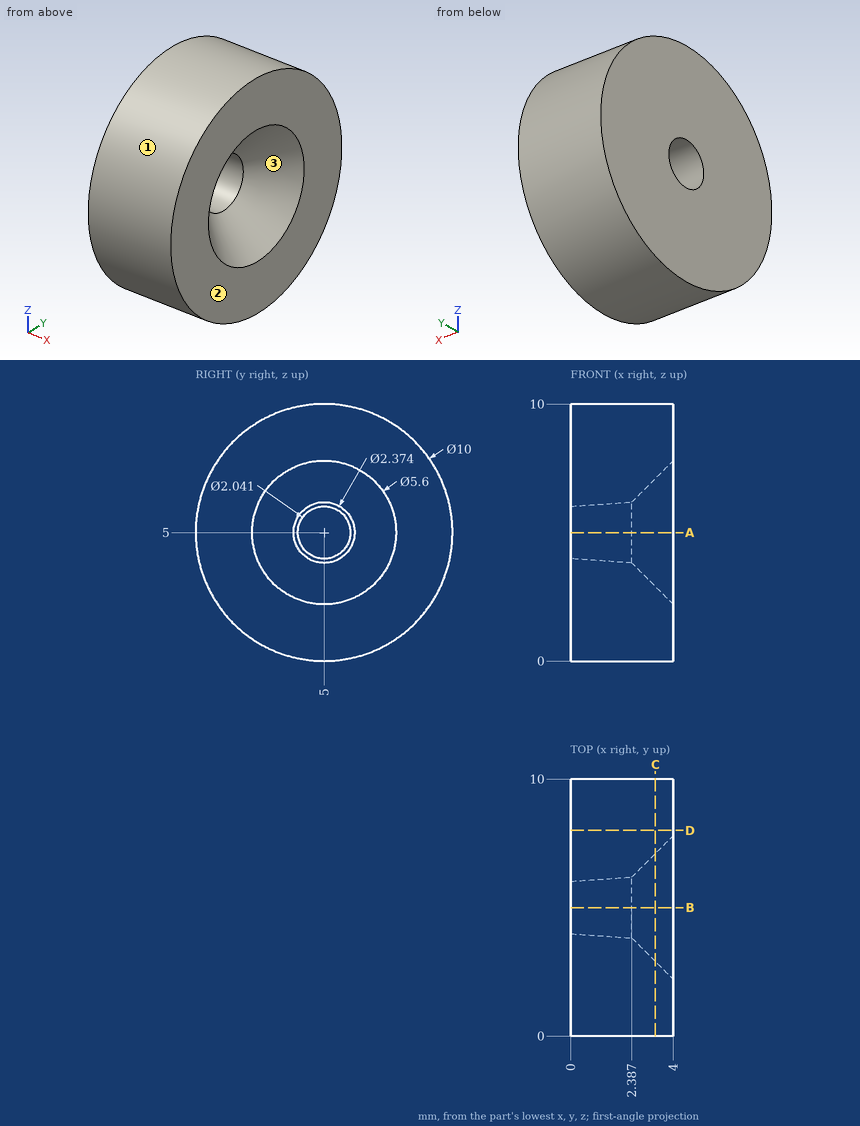
The drawing under review shows one solid part. Ordinate dimensions are in mm from its lowest x, y, z. Give positions to 0.01 mm unless a question says otherwise; leave off trailing zeros. Order: outer loops, then holes, each group sorted by start corner. A loop starts at its lowest first (then second) coordinate and runs counter-clockwise, first axis right, second up. Notation, with made-up numbers: (-23, 76) -> (1, 76) arc R35 ccw to (1, 111) -> close; hole circle Ø9 at (34, 5.5). An arc over 180 degrees is marked (long way). Write item = value, one per line. Start each with the question number.
(1) Mouldability with a two-part tool opening along Z and no side actions: class the marked faces 1, 2 and 3 as +Z half, -Z half, draft (parallel to the pull), parting line (faces both ways), or undercut.
(2) For pin 1 (1.5 mm diameter, centred on x = 1.5, y = 6.5, fed in from +Z), flat-tipped, find the tip position at first contact; note if it passes through.
(3) We need section D-D on y = 8. Write out the cut boundary in (x, z), plus the area to 3 significant figures.
(4) We need section C-C on x = 3.3. Write out the cut boundary in (y, z).
(5) To check wall thickness, follow line 1 along Z through (x, y) = (0.5, 5.5) (1 decimal); line 2 along Z through (x, y) = (3.7, 6.25) (1 decimal); line 3 along Y through (x, z) = (3.8, 3) (1 decimal). State the ranges of each line that lie inside material, in increasing order.
(6) We need section A-A on z = 5. Write out the cut boundary in (x, y), plus the area to 3 significant figures.
Numbers:
q1.face_1 = parting line
q1.face_2 = draft
q1.face_3 = undercut
q2.pin_1 = 9.94
q3.outline = (0, 1) -> (4, 1) -> (4, 9) -> (0, 9) -> close
q3.area = 32.0 mm^2
q4.outline = circle Ø10 at (5, 5); hole circle Ø4.2 at (5, 5)
q5.line_1 = 0 to 4.1, 5.9 to 10
q5.line_2 = 0.2 to 2.8, 7.2 to 9.8
q5.line_3 = 0.4 to 3.3, 6.7 to 9.6
q6.outline = (0, 0) -> (4, 0) -> (4, 2.2) -> (2.39, 3.81) -> (0, 3.98) -> close; (0, 6.02) -> (2.39, 6.19) -> (4, 7.8) -> (4, 10) -> (0, 10) -> close
q6.area = 28.3 mm^2
